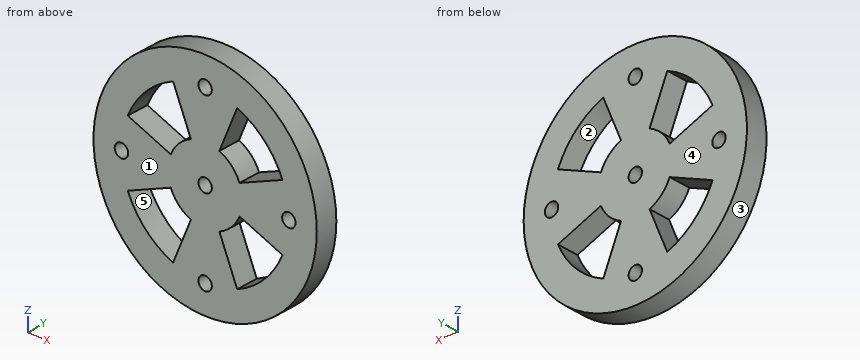
```python
from build123d import *

# Parameters (mm, degrees)
SKETCH1_R           = 25
SKETCH1_R_2         = 1.5
BOSS_EXTRUDE1_DEPTH = 5


with BuildPart() as part:
    # Sketch1 → Boss-Extrude1 (new body)
    with BuildSketch(Plane(origin=(0, 0, 0), x_dir=(1, 0, 0), z_dir=(0, 1, 0))):
        Circle(SKETCH1_R)
        Circle(SKETCH1_R_2, mode=Mode.SUBTRACT)
        with Locations((18.75, 0)):
            Circle(SKETCH1_R_2, mode=Mode.SUBTRACT)
        with Locations((0, -18.75)):
            Circle(SKETCH1_R_2, mode=Mode.SUBTRACT)
        with Locations((-18.75, 0)):
            Circle(SKETCH1_R_2, mode=Mode.SUBTRACT)
        with Locations((0, 18.75)):
            Circle(SKETCH1_R_2, mode=Mode.SUBTRACT)
        with BuildLine():
            Line((7.698996104, 3.189028603), (17.322741235, 7.175314357))
            ThreePointArc((17.322741235, 7.175314357), (13.258252147, 13.258252147), (7.175314357, 17.322741235))
            Line((7.175314357, 17.322741235), (3.189028603, 7.698996104))
            ThreePointArc((3.189028603, 7.698996104), (5.89255651, 5.89255651), (7.698996104, 3.189028603))
        make_face(mode=Mode.SUBTRACT)
        with BuildLine():
            Line((3.189028603, -7.698996104), (7.175314357, -17.322741235))
            ThreePointArc((7.175314357, -17.322741235), (13.258252147, -13.258252147), (17.322741235, -7.175314357))
            Line((17.322741235, -7.175314357), (7.698996104, -3.189028603))
            ThreePointArc((7.698996104, -3.189028603), (5.89255651, -5.89255651), (3.189028603, -7.698996104))
        make_face(mode=Mode.SUBTRACT)
        with BuildLine():
            Line((-7.698996104, -3.189028603), (-17.322741235, -7.175314357))
            ThreePointArc((-17.322741235, -7.175314357), (-13.258252147, -13.258252147), (-7.175314357, -17.322741235))
            Line((-7.175314357, -17.322741235), (-3.189028603, -7.698996104))
            ThreePointArc((-3.189028603, -7.698996104), (-5.89255651, -5.89255651), (-7.698996104, -3.189028603))
        make_face(mode=Mode.SUBTRACT)
        with BuildLine():
            Line((-7.698996104, 3.189028603), (-17.322741235, 7.175314357))
            ThreePointArc((-17.322741235, 7.175314357), (-13.258252147, 13.258252147), (-7.175314357, 17.322741235))
            Line((-7.175314357, 17.322741235), (-3.189028603, 7.698996104))
            ThreePointArc((-3.189028603, 7.698996104), (-5.89255651, 5.89255651), (-7.698996104, 3.189028603))
        make_face(mode=Mode.SUBTRACT)
    extrude(amount=BOSS_EXTRUDE1_DEPTH)


solid = part.part
```
Model file for the job. Use its own axes, mm. Face numbers are marked on the shaded views. A direction names the side the tool comes from. Round coordinates to 2 decimals unless told otherwise and drop trailing zeros. Write each loop counter-clockwise with the first axis right and the second up, starting at its lowest first coordinate (ties: lowest second). Pieces come first, ordered by that corner, then holes. Notation, with made-up numbers: (-5.75, 28) -> (50.25, 28) arc R13 cw to (50.25, 46) -> close; hole circle Ø9 at (-28, 79). An arc over 180 degrees is marked (long way). Answer as CSV lines item,"result".
1. Mould opens along X. For the marked faces 1, 2 and 3 say: +X half, -X half, draft (parallel to the pull), parting line (faces both ways), or undercut.
Resolved:
face 1,"draft"
face 2,"undercut"
face 3,"parting line"
2. Tool access for the marked faces 4 and 5: list every direction of +Z, -Z, +X, -X, +Y, -Y with a clear straight run to the whole face (end or side of a thin tool).
Resolved:
face 4,"+Z, -Z, +X, -X, +Y"
face 5,"+Y, -Y"
3. Pin check, flat tip, straight feed: pin 1 Ø3 at (x, y) = (18, 3.5) entering from +Z. Stop position of the tip, or through.
Resolved:
pin 1,"z = 18.78"
4. Slice it at A-A, the plane x = 0. List the corners of the cut face in (y, z).
Resolved:
outline,"(0, -25) -> (5, -25) -> (5, -20.25) -> (0, -20.25) -> close; (0, -17.25) -> (5, -17.25) -> (5, -1.5) -> (0, -1.5) -> close; (0, 1.5) -> (5, 1.5) -> (5, 17.25) -> (0, 17.25) -> close; (0, 20.25) -> (5, 20.25) -> (5, 25) -> (0, 25) -> close"
5. Slice it at C-C, the plane y = 2.05. State how many separate pieces and enclosed holes the cut face has, plus the area to 4 significant figures.
Resolved:
separate pieces,"1"
enclosed holes,"9"
area,"1,485 mm²"
6. Slice it at D-D, the plane z = 0. List the corners of the cut face in (x, y).
Resolved:
outline,"(-25, 0) -> (-20.25, 0) -> (-20.25, 5) -> (-25, 5) -> close; (-17.25, 0) -> (-1.5, 0) -> (-1.5, 5) -> (-17.25, 5) -> close; (1.5, 0) -> (17.25, 0) -> (17.25, 5) -> (1.5, 5) -> close; (20.25, 0) -> (25, 0) -> (25, 5) -> (20.25, 5) -> close"
7. Drill centre lines: line 1 (Z direction, x = 0, y = 2.45); line 2 (X direction, y = 3.75, z = 5). Where is each one in solid material? Low to high.
Resolved:
line 1,"-25 to -20.25, -17.25 to -1.5, 1.5 to 17.25, 20.25 to 25"
line 2,"-24.49 to -12.07, -6.67 to 6.67, 12.07 to 24.49"
8. Slice it at B-B, the plane z = 13. List the corners of the cut face in (x, y).
Resolved:
outline,"(-21.35, 0) -> (-13.51, 0) -> (-13.51, 5) -> (-21.35, 5) -> close; (-5.38, 0) -> (5.38, 0) -> (5.38, 5) -> (-5.38, 5) -> close; (13.51, 0) -> (21.35, 0) -> (21.35, 5) -> (13.51, 5) -> close"
